```python
from build123d import *

# Parameters (mm, degrees)
CROQUIS1_W              = 100
CROQUIS1_H              = 85
SALIENTE_EXTRUIR1_DEPTH = 20
CORTAR_EXTRUIR1_REACH   = 102
CORTAR_EXTRUIR2_REACH   = 102
CORTAR_EXTRUIR6_DEPTH   = 5
CROQUIS11_W             = 15
CROQUIS11_H             = 16
CORTAR_EXTRUIR7_DEPTH   = 44
CROQUIS12_W             = 5
CROQUIS12_H             = 49.877192982
CORTAR_EXTRUIR8_DEPTH   = 44
CORTAR_EXTRUIR9_REACH   = 97
CROQUIS13_W             = 50
CROQUIS13_H             = 18
CROQUIS14_W             = 9.804862201
CROQUIS14_H             = 2
CORTAR_EXTRUIR10_DEPTH  = 121
CORTAR_EXTRUIR11_REACH  = 97
CORTAR_EXTRUIR12_REACH  = 97
CORTAR_EXTRUIR13_DEPTH  = 96


with BuildPart() as part:
    # Croquis1 → Saliente-Extruir1 (new body)
    with BuildSketch(Plane(origin=(0, 0, 0), x_dir=(1, 0, 0), z_dir=(0, 1, 0))):
        with Locations((-9.795321637, 18.377192982)):
            Rectangle(CROQUIS1_W, CROQUIS1_H)
    extrude(amount=SALIENTE_EXTRUIR1_DEPTH)

    # Croquis3 → Cortar-Extruir1 (cut, up to next)
    with BuildSketch(Plane(origin=(40.204678363, 0, 0), x_dir=(0, 0, -1), z_dir=(1, 0, 0)), mode=Mode.PRIVATE) as cortar_extruir1_sk1:
        Polygon((-24.122807018, 0), (0.976475977, 20), (-24.122807018, 20), align=None)
    cortar_extruir1_tool1 = extrude(cortar_extruir1_sk1.sketch, amount=-CORTAR_EXTRUIR1_REACH, mode=Mode.PRIVATE) & part.part
    add(cortar_extruir1_tool1.solids().sort_by_distance((40.204678, 13.333333, 15.756379))[0], mode=Mode.SUBTRACT)

    # Croquis4 → Cortar-Extruir2 (cut, up to next)
    with BuildSketch(Plane(origin=(40.204678363, 0, 0), x_dir=(0, 0, -1), z_dir=(1, 0, 0)), mode=Mode.PRIVATE) as cortar_extruir2_sk1:
        Polygon((0.976475977, 20), (0.976475977, 15), (-24.122807018, 0), align=None)
    cortar_extruir2_tool1 = extrude(cortar_extruir2_sk1.sketch, amount=-CORTAR_EXTRUIR2_REACH, mode=Mode.PRIVATE) & part.part
    add(cortar_extruir2_tool1.solids().sort_by_distance((40.204678, 11.666667, 7.389952))[0], mode=Mode.SUBTRACT)

    # Croquis8 → Cortar-Extruir6 (cut)
    with BuildSketch(Plane.ZY.offset(59.795321637)):
        Polygon((-11, 20), (-0.976475977, 20), (-0.976475977, 15), (24.122807018, 0), (-11, 0), align=None)
    extrude(amount=-CORTAR_EXTRUIR6_DEPTH, mode=Mode.SUBTRACT)

    # Croquis11 → Cortar-Extruir7 (cut)
    with BuildSketch(Plane.XY.offset(-11)):
        with Locations((27.704678363, 12)):
            Rectangle(CROQUIS11_W, CROQUIS11_H)
        Polygon((0.204678363, 20), (-14.795321637, 20), (-14.795321637, 4), (0.204678363, 4), (0.204678363, 18.881828366), align=None)
        with Locations((-42.295321637, 12)):
            Rectangle(CROQUIS11_W, CROQUIS11_H)
    extrude(amount=CORTAR_EXTRUIR7_DEPTH, mode=Mode.SUBTRACT)

    # Croquis12 → Cortar-Extruir8 (cut)
    with BuildSketch(Plane(origin=(0, 20, 0), x_dir=(1, 0, 0), z_dir=(0, 1, 0))):
        with Locations((-57.295321637, 35.938596491)):
            Rectangle(CROQUIS12_W, CROQUIS12_H)
    extrude(amount=-CORTAR_EXTRUIR8_DEPTH, mode=Mode.SUBTRACT)

    # Croquis13 → Cortar-Extruir9 (cut, up to next)
    with BuildSketch(Plane(origin=(40.204678363, 0, 0), x_dir=(0, 0, -1), z_dir=(1, 0, 0)), mode=Mode.PRIVATE) as cortar_extruir9_sk1:
        with Locations((35.877192982, 11)):
            Rectangle(CROQUIS13_W, CROQUIS13_H)
    cortar_extruir9_tool1 = extrude(cortar_extruir9_sk1.sketch, amount=-CORTAR_EXTRUIR9_REACH, mode=Mode.PRIVATE) & part.part
    add(cortar_extruir9_tool1.solids().sort_by_distance((40.204678, 11, -35.877193))[0], mode=Mode.SUBTRACT)

    # Croquis14 → Cortar-Extruir10 (cut)
    with BuildSketch(Plane(origin=(40.204678363, 0, 0), x_dir=(0, 0, -1), z_dir=(1, 0, 0))):
        with Locations((5.779624083, 1)):
            Rectangle(CROQUIS14_W, CROQUIS14_H)
    extrude(amount=-CORTAR_EXTRUIR10_DEPTH, mode=Mode.SUBTRACT)

    # Croquis17 → Cortar-Extruir11 (cut, up to next)
    with BuildSketch(Plane(origin=(40.204678363, 0, 0), x_dir=(0, 0, -1), z_dir=(1, 0, 0)), mode=Mode.PRIVATE) as cortar_extruir11_sk1:
        Polygon((10.877192982, 2), (10.682055183, 0), (60.877192982, 0), (60.877192982, 2), align=None)
    cortar_extruir11_tool1 = extrude(cortar_extruir11_sk1.sketch, amount=-CORTAR_EXTRUIR11_REACH, mode=Mode.PRIVATE) & part.part
    add(cortar_extruir11_tool1.solids().sort_by_distance((40.204678, 0.999351, -35.828377))[0], mode=Mode.SUBTRACT)

    # Croquis18 → Cortar-Extruir12 (cut, up to next)
    with BuildSketch(Plane(origin=(40.204678363, 0, 0), x_dir=(0, 0, -1), z_dir=(1, 0, 0)), mode=Mode.PRIVATE) as cortar_extruir12_sk1:
        Polygon((10.682055183, 2), (10.877192982, 2), (10.682055183, 0), align=None)
    cortar_extruir12_tool1 = extrude(cortar_extruir12_sk1.sketch, amount=-CORTAR_EXTRUIR12_REACH, mode=Mode.PRIVATE) & part.part
    add(cortar_extruir12_tool1.solids().sort_by_distance((40.204678, 1.333333, -10.747101))[0], mode=Mode.SUBTRACT)

    # Croquis19 → Cortar-Extruir13 (cut)
    with BuildSketch(Plane.ZY.offset(54.795321637)):
        Polygon((-0.976475977, 15), (-5.92683448, 20), (-0.976475977, 20), align=None)
    extrude(amount=-CORTAR_EXTRUIR13_DEPTH, mode=Mode.SUBTRACT)


solid = part.part
```
CAD build for the part. Positions are in the model's coordinates, mm. A direction names the side the tool comes from. Coordinates: 2 decimals unless noted, no trailing zeros. Loops run counter-clockwise (first coordinate to the right, second up) from the corner with the lowest first, then second, coordinate; pieces in that order, holes last. Notation, with made-up numbers: (89.5, 64) - (129.5, 64) arc R26 ccw to (129.5, 101) - close; hole circle Ø8 at (42, 62). An arc over 180 degrees is marked (long way). Return JSON: item names as keys, results as strings.
1. Band-saw the part on C-C (x = -32). Give the cut face in (y, z), and give its area (3 significant figures).
Result:
{"outline": "(0, -0.88) - (2, -0.88) - (2, -10.88) - (20, -10.88) - (20, -5.93) - (15, -0.98) - (0, 24.12) - close", "area": "354 mm2"}
2. Probe L1, parallel to X at y = 10.25, z = -3; L2, parallel to Y at x = 29, z = 5.5; L3, parallel to Z at x = -31, y = 7. List the from-to ranges inside material, lowest first. Write a range as from..to.
Result:
{"L1": "x = -54.8..-49.8, -34.8..-14.8, 0.2..20.2, 35.2..40.2", "L2": "y = 0..4", "L3": "z = -10.88..12.41"}
3. Drop flat-ended pins along their axis: pin 1 (1.6 mm diameter, centred on x = -3, y = 1, fed in from -Z); pin 2 (3 mm diameter, centred on x = -11.5, z = -1.5, fed in from -Y); pin 3 (11 mm diameter, centred on x = -9, z = -7, fed in from -Y); pin 4 (12 mm diameter, centred on x = 29.5, z = 5, fed in from +Y). Give the stop position or say it passes through.
Result:
{"pin 1": "stops at z = -0.88", "pin 2": "stops at y = 0", "pin 3": "stops at y = 2", "pin 4": "stops at y = 12.54"}
4. Mould opens along X. For faces 1 (the flat face through (-54.795, 8, -1)), 2 (the flat face through (-24.935, 17.465, -3.417)), 3 (the flat face through (40.205, 8, 3)), 4 (the flat face through (-34.795, 10, 0)) say: released by +X, released by -X, zero draft, split by the parting line, or undercut.
Result:
{"face 1": "released by -X", "face 2": "zero draft", "face 3": "released by +X", "face 4": "undercut"}
5. Band-saw the part on A-A (y = 8.75). Give the cut face in (x, z).
Result:
{"outline": "(-54.8, -10.88) - (-49.8, -10.88) - (-49.8, 9.48) - (-54.8, 9.48) - close; (-34.8, -10.88) - (-14.8, -10.88) - (-14.8, 9.48) - (-34.8, 9.48) - close; (0.2, -10.88) - (20.2, -10.88) - (20.2, 9.48) - (0.2, 9.48) - close; (35.2, -10.88) - (40.2, -10.88) - (40.2, 9.48) - (35.2, 9.48) - close"}
6. Band-saw the part on D-D (y = 5). Give the cut face in (x, z).
Result:
{"outline": "(-54.8, -10.88) - (-49.8, -10.88) - (-49.8, 15.76) - (-54.8, 15.76) - close; (-34.8, -10.88) - (-14.8, -10.88) - (-14.8, 15.76) - (-34.8, 15.76) - close; (0.2, -10.88) - (20.2, -10.88) - (20.2, 15.76) - (0.2, 15.76) - close; (35.2, -10.88) - (40.2, -10.88) - (40.2, 15.76) - (35.2, 15.76) - close"}
7. 3-axis set-ups, long thin cutter, end or side, ignore diameter. For faces 5 (the flat face through (28, 4, 3)), 6 (the flat face through (-52.33, 17.465, -3.417)), 7 (the flat face through (-7, 2, -6)): which of +Z, -Z, +X, -X, +Y, -Y reach the whole face in a straight line?
Result:
{"face 5": "+Z, -Z, +Y", "face 6": "+Z, +X, -X, +Y", "face 7": "-Z, +X, -X, -Y"}
8. Band-saw the part on B-B (z = -8.5). Give the cut face in (x, y), and give its area (3 significant figures).
Result:
{"outline": "(-54.8, 2) - (40.2, 2) - (40.2, 20) - (35.2, 20) - (35.2, 4) - (20.2, 4) - (20.2, 20) - (0.2, 20) - (0.2, 4) - (-14.8, 4) - (-14.8, 20) - (-34.8, 20) - (-34.8, 4) - (-49.8, 4) - (-49.8, 20) - (-54.8, 20) - close", "area": "990 mm2"}
